```python
from build123d import *

# Parameters (mm, degrees)
F0_W     = 460
F0_H     = 650
F1_DEPTH = 90
F2_W     = 420
F2_H     = 70
F3_DEPTH = 650.001
F4_W     = 600
F4_H     = 2.5
F5_DEPTH = 460.001
F7_D     = 5
F7_DEPTH = 20.001
F9_D     = 5.5
F9_DEPTH = 20.001


with BuildPart() as f1:
    # F0 (on Top) → F1 (new body)
    with BuildSketch(Plane.XY):
        Rectangle(F0_W, F0_H)
    extrude(amount=F1_DEPTH)

    # F2 (on face) → F3 (cut, through all)
    with BuildSketch(Plane.XZ.offset(325)):
        with Locations((0, 35)):
            Rectangle(F2_W, F2_H)
    extrude(amount=-F3_DEPTH, mode=Mode.SUBTRACT)

    # F4 (on face) → F5 (cut, through all)
    with BuildSketch(Plane.YZ.offset(230)):
        with Locations((-25, 31.25)):
            Rectangle(F4_W, F4_H)
    extrude(amount=-F5_DEPTH, mode=Mode.SUBTRACT)

    # F7 (through all, one way)
    with BuildSketch(Plane.YZ.offset(-210)):
        with Locations((-305, 10), (305, 10)):
            Circle(F7_D / 2)
    extrude(amount=-F7_DEPTH, mode=Mode.SUBTRACT)

    # F9 (through all, one way)
    with BuildSketch(Plane(origin=(210, 0, 0), x_dir=(0, -1, 0), z_dir=(-1, 0, 0))):
        with Locations((305, 10), (-305, 10)):
            Circle(F9_D / 2)
    extrude(amount=-F9_DEPTH, mode=Mode.SUBTRACT)


solid = f1.part
```
Geometry: final body of the model. Coordinates: model frame, mm. A direction names the side the tool comes from. Give positions to 0.01 mm unless a question says otherwise; leave off trailing zeros. Loops run counter-clockwise (first coordinate to the right, second up) from the corner with the lowest first, then second, coordinate; pieces in that order, holes last. Notation, with made-up numbers: (-17, 78.25) -> (2, 78.25) arc R21 ccw to (2, 92.25) -> close; hole circle Ø5 at (8, 33). An arc over 180 degrees is marked (long way). Use one line per item in the form item = value.
Item 1: Section query C-C on x = 102.5. Output: boundary loops of the cut face in (y, z).
A:
outline = (-325, 70) -> (325, 70) -> (325, 90) -> (-325, 90) -> close
Item 2: Section query B-B on y = -261. Output: boundary loops of the cut face in (x, z).
A:
outline = (-230, 0) -> (-210, 0) -> (-210, 30) -> (-230, 30) -> close; (-230, 32.5) -> (-210, 32.5) -> (-210, 70) -> (210, 70) -> (210, 32.5) -> (230, 32.5) -> (230, 90) -> (-230, 90) -> close; (210, 0) -> (230, 0) -> (230, 30) -> (210, 30) -> close
Item 3: Line query: probe 1 along Z at (x, y) = (225, -305); probe 2 along Z at (x, y) = (-218, -305); probe 3 along X at (y, z) = (-119, 11.5). Output: solid intervals per line, ascending.
A:
probe_1 = 0 to 7.25, 12.75 to 30, 32.5 to 90
probe_2 = 0 to 7.5, 12.5 to 30, 32.5 to 90
probe_3 = -230 to -210, 210 to 230
Item 4: Access query for faces 4 (the face through (-3, -5, 70)), 5 (the face through (-220, -29, 32.5)), 6 (the face through (-230, -5, 44)). Directions: +Z, -Z, +X, -X, +Y, -Y. A direction counts if a zero-diameter tool reaches every point of the face in a straight line with its end or side. Return the directions, or none.
A:
face_4 = -Z, +Y, -Y
face_5 = +X, -X, -Y
face_6 = +Z, -Z, -X, +Y, -Y
Item 5: Section query A-A on z = 51. Output: boundary loops of the cut face in (x, y), and give its area (3 significant figures).
A:
outline = (-230, -325) -> (-210, -325) -> (-210, 325) -> (-230, 325) -> close; (210, -325) -> (230, -325) -> (230, 325) -> (210, 325) -> close
area = 26,000 mm^2
Item 6: Pin query (flat end, axial travel): P1, Ø6, axis at x = 134.5, y = -158.5, coming from the -Z side. Return the tip coordinate at first contact, or that it passes through.
A:
P1 = 70
Item 7: Draft query along Z for faces 1 (the face through (-220, 5, 0)), 2 (the face through (-210, -5, 35)), 3 (the face through (220, -29, 30)). Return one class per face: pulls with the +Z half, pulls with the -Z half, needs draft (parallel to the pull), parting line crosses it, or undercut.
A:
face_1 = pulls with the -Z half
face_2 = needs draft
face_3 = undercut
